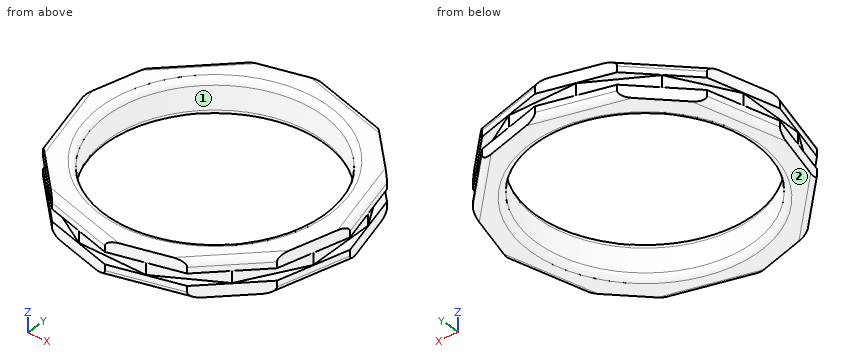
```python
from build123d import *

# Parameters (mm, degrees)
F2_DEPTH = 0.5
F4_DEPTH = 1
F0_R     = 9.1
F6_DEPTH = 2.5
F7_R     = 0.5
F8_R     = 0.5


with BuildPart() as f2:
    # F1 (on Top) → F2 (new body, symmetric)
    with BuildSketch(Plane.XY):
        Polygon((-10.6, -2.8402614398), (-7.7597385602, -7.7597385602), (-2.8402614398, -10.6), (2.8402614398, -10.6), (7.7597385602, -7.7597385602), (10.6, -2.8402614398), (10.6, 2.8402614398), (7.7597385602, 7.7597385602), (2.8402614398, 10.6), (-2.8402614398, 10.6), (-7.7597385602, 7.7597385602), (-10.6, 2.8402614398), align=None)
    extrude(amount=F2_DEPTH, both=True)

    # F3 (on face) → F4 (join)
    with BuildSketch(Plane.XY.offset(0.5)):
        Polygon((-9.8623301938, 5.6940189923), (-11.3880379845, 0), (-9.8623301938, -5.6940189923), (-5.6940189923, -9.8623301938), (0, -11.3880379845), (5.6940189923, -9.8623301938), (9.8623301938, -5.6940189923), (11.3880379845, 0), (9.8623301938, 5.6940189923), (5.6940189923, 9.8623301938), (0, 11.3880379845), (-5.6940189923, 9.8623301938), align=None)
    extrude(amount=F4_DEPTH)

    # F5: F2 across plane


with BuildPart() as f2_1:
    add(f2.part)
    add(f2.part.mirror(Plane.XY))

    # F0 (on Top) → F6 (cut, symmetric)
    with BuildSketch(Plane.XY):
        Circle(F0_R)
    extrude(amount=F6_DEPTH, both=True, mode=Mode.SUBTRACT)

    # F7
    f7_edges = [f2_1.edges().sort_by_distance(p)[0] for p in [
        (-9.1, 0, -1.5),
        (9.1, 0, 0),
        (-9.1, 0, 1.5),
    ]]
    fillet(f7_edges, radius=F7_R)

    # F8
    f8_edges = [f2_1.edges().sort_by_distance(p)[0] for p in [
        (10.625184, -2.847009, -1.5),
        (7.778175, 7.778175, -1.5),
        (-2.847009, 10.625184, -1.5),
        (-10.625184, 2.847009, -1.5),
        (-7.778175, -7.778175, -1.5),
        (2.847009, -10.625184, -1.5),
        (-2.847009, -10.625184, 1.5),
        (7.778175, -7.778175, 1.5),
        (10.625184, 2.847009, 1.5),
        (2.847009, 10.625184, 1.5),
        (-7.778175, 7.778175, 1.5),
        (-10.625184, -2.847009, 1.5),
    ]]
    fillet(f8_edges, radius=F8_R)


solid = f2_1.part
```
Check sheet for the modelled part. Datum: model origin and axes. Units: mm. Face numbers are marked on the shaded views. Round coordinates to 2 decimals unless told otherwise and drop trailing zeros. Order: outer loops, then holes, each group sorted by start corner. A loop starts at its lowest first (then second) coordinate and runs counter-clockwise, first axis right, second up. Notation, with made-up numbers: (89.25, 59) -> (116.25, 59) arc R30 ccw to (116.25, 93) -> close; hole circle Ø10 at (-14, 23.5). An arc over 180 degrees is marked (long way). Use CSV: the item, a comma, the result in double quotes.
(1) Cross-section at A-A (z = 0.15). Record the boundary of the cut face in (x, y), and give its area (3 significant figures).
Worked out:
outline,"(-10.6, -2.84) -> (-7.76, -7.76) -> (-2.84, -10.6) -> (2.84, -10.6) -> (7.76, -7.76) -> (10.6, -2.84) -> (10.6, 2.84) -> (7.76, 7.76) -> (2.84, 10.6) -> (-2.84, 10.6) -> (-7.76, 7.76) -> (-10.6, 2.84) -> close; hole circle Ø18.2 at (0, 0)"
area,"101 mm²"
(2) Draft check along Y on the marked faces 1 and 2. Enter one of: pulls with the +Y half, pulls with the -Y half, needs draft (parallel to the pull), parting line crosses it, or undercut.
Worked out:
face 1,"undercut"
face 2,"needs draft"
(3) Depth check by flat-ended pin: pin 1 (0.8 mm diameter, centred on y = 0.5, z = 0, fed in from -X); pin 2 (0.5 mm diameter, centred on x = 0, z = 0, fed in from -Y); pin 3 (0.8 mm diameter, centred on y = 1.5, z = 0, fed in from +X). Enter the tip coordinate at first touch or a pass-through.
Worked out:
pin 1,"x = -10.6"
pin 2,"y = -10.6"
pin 3,"x = 10.6"
(4) Material ranges on line 1 along Y through (x, z) = (0, 0); line 2 along Y through (x, z) = (6.25, 1.35); line 3 along X through (y, z) = (-7.5, 0.15), recorded low to high. Write a range as from..to.
Worked out:
line 1,"-10.6..-9.1, 9.1..10.6"
line 2,"-9.1..-6.81, 6.81..9.31"
line 3,"-7.91..-5.15, 5.15..7.91"
